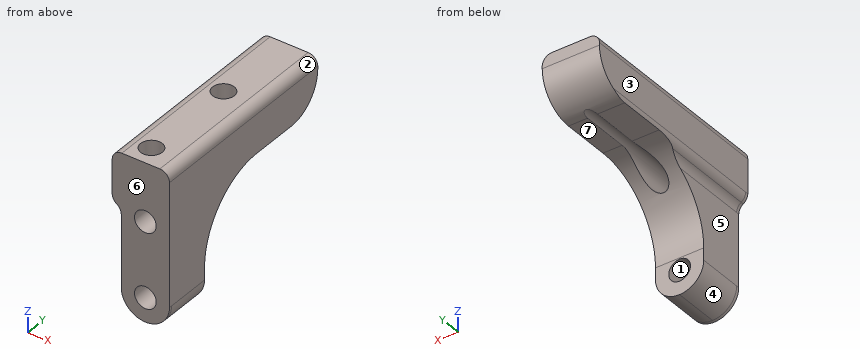
Autodesk Inventor part; units mm, degrees
ref_plane "YZ Plane" through (0, 0, 0) normal (1, 0, 0) x (0, 1, 0)
ref_plane "XZ Plane" through (0, 0, 0) normal (0, 1, 0) x (-1, 0, 0)
ref_plane "XY Plane" through (0, 0, 0) normal (0, 0, 1) x (1, 0, 0)
sketch "スケッチ1" plane through (0, 0, 0) normal (0, 0, 1) x (1, 0, 0)
  line L0 (0, 0) -> (25.5, 0)
  line L1 (25.5, 0) -> (25.5, 41.76)
  line L2 (25.5, 41.76) -> (0, 41.76)
  line L3 (0, 41.76) -> (0, 0)
  line L4 (0, 3) -> (25.5, 3) construction
  line L5 (13.5, 41.76) -> (13.5, 0) construction
  line L6 (12, 41.76) -> (12, 0) construction
  line L7 (12, 7.267) -> (13.5, 7.267)
  line L8 (13.5, 7.267) -> (13.5, 17.554)
  line L9 (13.5, 17.554) -> (12, 17.554)
  line L10 (12, 17.554) -> (12, 7.267)
  line L11 (12, 27.612) -> (13.5, 27.612)
  line L12 (13.5, 27.612) -> (13.5, 37.899)
  line L13 (13.5, 37.899) -> (12, 37.899)
  line L14 (12, 37.899) -> (12, 27.612)
  dimension "d0" = 3
  dimension "d1" = 38.76
  dimension "d2" = 1.5
  dimension "d3" = 12
  dimension "d4" = 25.5
  dimension "d5" = 4.267
  dimension "d6" = 10.287
  dimension "d7" = 10.058
  dimension "d8" = 10.287
  dimension "d11" = 12
extrude "押し出し1" add sketch "スケッチ1" along normal mid plane 7.5
sketch "スケッチ2" plane through (0, 0, -3.75) normal (0, -1, 0) x (1, 0, 0)
  line L0 (25.5, 7.5) -> (0, 7.5)
  line L1 (0, 7.5) -> (25.5, 7.5)
  line L2 (25.5, 7.5) -> (25.5, 2.5)
  line L3 (25.5, -2.5) -> (20.5, -2.5)
  line L4 (0, -2.5) -> (0, 2.5)
  line L5 (25.5, 2.5) -> (0, 2.5) construction
  line L6 (0, 3.75) -> (0, 7.5) construction
  arc A0 (0, 2.5) -> (5, -2.5) centre (5, 2.5) ccw
  line L7 (5, 2.5) -> (5, -2.5) construction
  line L8 (5, 2.5) -> (0, 2.5) construction
  arc A1 (20.5, -2.5) -> (25.5, 2.5) centre (20.5, 2.5) ccw
  line L9 (20.5, 2.5) -> (20.5, -2.5) construction
  line L10 (20.5, 2.5) -> (25.5, 2.5) construction
  line L11 (25.5, 0) -> (25.5, 7.5)
  line L12 (0, 2.5) -> (0, 7.5)
  line L13 (5, -2.5) -> (0, -2.5)
  line L14 (20.5, -2.5) -> (5, -2.5)
  line L15 (25.5, 2.5) -> (25.5, -2.5)
  dimension "d12" = 90
  dimension "d13" = 90
  dimension "d14" = 10
  dimension "d15" = 5
extrude "押し出し2" add sketch "スケッチ2" against normal up to surface (7.267 mm away)
extrude "押し出し3" [suppressed]
ref_plane "作業平面1" through (0, 0, -1.25) normal (0, 0, 1) x (1, 0, 0)
sketch "スケッチ3" plane through (0, 0, 3.75) normal (0, -1, 0) x (1, 0, 0)
  arc A0 (0, -5) -> (5, -10) centre (5, -5) ccw construction
  arc A1 (20.5, -10) -> (25.5, -5) centre (20.5, -5) ccw construction
  circle A2 centre (5, -5) radius 2.25
  circle A3 centre (20.5, -5) radius 2.25
  point P0 (0, -3.75)
  dimension "d20" = 4.5
  dimension "d21" = 4.5
extrude "押し出し4" cut sketch "スケッチ3" against normal up to surface (41.76 mm away)
sketch "スケッチ4" plane through (0.6699, 41.76, -3.75) normal (0, 1, 0) x (1, 0, 0)
  circle A0 centre (19.8301, -2.5) radius 2.25 construction
  circle A1 centre (4.3301, -2.5) radius 2.25 construction
  line L0 (0, 0) -> (24.1603, 0)
  line L1 (19.8301, 0) -> (19.8301, -2.5) construction
  line L2 (17.5801, 0) -> (17.5801, -2.5)
  line L3 (22.0801, -2.5) -> (22.0801, 0)
  arc A2 (22.0801, 0) -> (17.5801, 0) centre (19.8301, 0) ccw
  arc A3 (17.5801, -2.5) -> (22.0801, -2.5) centre (19.8301, -2.5) ccw
  line L4 (4.3301, -0.25) -> (4.3301, -2.5) construction
  line L5 (2.0801, -0.25) -> (2.0801, -2.5)
  line L6 (6.5801, -2.5) -> (6.5801, -0.25)
  arc A4 (6.5801, -0.25) -> (2.0801, -0.25) centre (4.3301, -0.25) ccw
  arc A5 (2.0801, -2.5) -> (6.5801, -2.5) centre (4.3301, -2.5) ccw
  point P0 (-0.6699, -3.75)
  point P1 (19.8301, -1.25)
  point P2 (4.3301, -1.375)
extrude "押し出し5" [suppressed]
sketch "スケッチ5" plane through (12, 7.267, 3.75) normal (1, 0, 0) x (0, 0, -1)
  line L0 (0, 0) -> (7.5, 0) construction
  line L1 (7.5, 10.287) -> (0, 10.287) construction
  line L2 (7.5, 10.287) -> (10, 12.787)
  line L3 (10, 12.787) -> (10, -2.5)
  line L4 (10, -2.5) -> (7.5, 0)
  line L5 (7.5, 0) -> (7.5, 10.287)
  line L6 (10, -7.267) -> (10, 0)
  point P0 (3.75, -7.267)
  dimension "d28" = 135
  dimension "d29" = 135
sketch "スケッチ6" plane through (0, 0, 3.75) normal (0, 0, 1) x (1, 0, 0)
  line L0 (12, 27.612) -> (12, 37.899) construction
  line L1 (12, 37.899) -> (13.5, 37.899) construction
  line L2 (13.5, 37.899) -> (13.5, 27.612) construction
  line L3 (13.5, 27.612) -> (12, 27.612) construction
  line L4 (12, 7.267) -> (12, 17.554) construction
  line L5 (12, 17.554) -> (13.5, 17.554) construction
  line L6 (13.5, 17.554) -> (13.5, 7.267) construction
  line L7 (13.5, 7.267) -> (12, 7.267) construction
  line L8 (0, 0) -> (25.5, 0) construction
  line L9 (25.5, 41.76) -> (0, 41.76) construction
  line L10 (13.625, 27.487) -> (13.625, 38.024)
  line L11 (13.625, 38.024) -> (11.875, 38.024)
  line L12 (11.875, 38.024) -> (11.875, 27.487)
  line L13 (11.875, 27.487) -> (13.625, 27.487)
  line L14 (13.625, 7.142) -> (13.625, 17.679)
  line L15 (13.625, 17.679) -> (11.875, 17.679)
  line L16 (11.875, 17.679) -> (11.875, 7.142)
  line L17 (11.875, 7.142) -> (13.625, 7.142)
  line L18 (0, 41.76) -> (0, 0)
  line L19 (25.5, 0) -> (25.5, 41.76)
  dimension "d32" = 0.125
  dimension "d33" = 0.125
extrude "押し出し7" cut sketch "スケッチ6" against normal through all
sketch "スケッチ8" plane through (0, 0, 3.75) normal (0, -1, 0) x (1, 0, 0)
  line L0 (13.625, 0) -> (13.625, -10) construction
  line L1 (0, 0) -> (0, -10)
  line L2 (0, 0) -> (13.625, 0)
  line L3 (13.625, 0) -> (13.625, -10)
  line L4 (13.625, -10) -> (0, -10)
  line L5 (0, -10) -> (0, 0)
  point P0 (0, -3.75)
extrude "押し出し10" cut sketch "スケッチ8" against normal up to surface (41.76 mm away)
sketch "スケッチ9" plane through (25.5, 7.267, -3.75) normal (0, 1, 0) x (1, 0, 0)
  line L0 (-11.875, 2.5) -> (-11.875, 0)
  line L1 (0, 0) -> (-11.875, 0)
  line L2 (0, 0) -> (0, 2.5)
  line L3 (0, 2.5) -> (-11.875, 2.5)
  point P0 (-25.5, -3.75)
extrude "押し出し11" add sketch "スケッチ9" along normal up to surface (34.493 mm away)
sketch "スケッチ10" plane through (25.5, 0, -6.25) normal (0, -1, 0) x (1, 0, 0)
  line L0 (-11.875, 0) -> (0, 0)
  line L1 (-11.875, 0) -> (0, 0)
  line L2 (0, 0) -> (0, -22.5)
  line L3 (0, -22.5) -> (-11.875, -22.5)
  line L4 (-11.875, -22.5) -> (-11.875, 0)
  circle A0 centre (-5, 5) radius 2.25 construction
  line L5 (-5, 5) -> (-5, -17.5) construction
  circle A1 centre (-5, -17.5) radius 2.25
  point P0 (-25.5, 6.25)
  dimension "d46" = 22.5
  dimension "d47" = 5
  dimension "d48" = 5
extrude "押し出し12" add sketch "スケッチ10" against normal up to surface (41.76 mm away)
sketch "スケッチ12" plane through (13.625, 0, 3.75) normal (0, -1, 0) x (1, 0, 0)
  circle A0 centre (6.875, -5) radius 2.25
  point P0 (-13.625, -3.75)
extrude "押し出し14" add sketch "スケッチ12" against normal up to surface (41.76 mm away)
sketch "スケッチ11" plane through (0, 0, 3.75) normal (0, 0, 1) x (1, 0, 0)
  line L0 (22.75, 0) -> (18.25, 0) construction
  line L1 (18.723, 0) -> (18.723, 3.589) construction
  circle A0 centre (18.723, 3.589) radius 2.25
  line L2 (13.625, 41.76) -> (13.625, 0)
  line L3 (18.723, 3.589) -> (18.723, 24.163) construction
  line L4 (18.25, 0) -> (18.25, 41.76) construction
  circle A1 centre (18.723, 24.163) radius 2.25
  point P0 (0, 0)
  dimension "d51" = 4.5
  dimension "d52" = 3.589
  dimension "d53" = 5.098
  dimension "d54" = 20.574
extrude "押し出し13" cut sketch "スケッチ11" against normal blind 7.5
sketch "スケッチ13" plane through (13.625, 0, 3.75) normal (0, -1, 0) x (1, 0, 0)
  circle A0 centre (6.875, -27.5) radius 2.25 construction
  line L0 (6.875, -27.5) -> (6.875, -12) construction
  circle A1 centre (6.875, -12) radius 2.25
  point P0 (-13.625, -3.75)
  dimension "d59" = 15.5
extrude "押し出し15" cut sketch "スケッチ13" against normal up to surface (41.76 mm away)
sketch "スケッチ14" plane through (13.625, 0, 3.75) normal (0, -1, 0) x (1, 0, 0)
  line L0 (2.848, -7.5) -> (7.348, -7.5) construction
  line L1 (2.848, 0) -> (7.348, 0) construction
  line L2 (0, -32.5) -> (0, 0)
  line L3 (0, -32.5) -> (1.875, -32.5)
  line L4 (1.875, -32.5) -> (1.875, -10.5)
  line L5 (1.875, -10.5) -> (0, -10.5)
  line L6 (0, -10.5) -> (0, -32.5)
  circle A0 centre (6.875, -27.5) radius 2.25
  point P0 (-13.625, -3.75)
  dimension "d62" = 3
  dimension "d63" = 5
extrude "押し出し16" cut sketch "スケッチ14" against normal up to surface (41.76 mm away) contours L2 L5 L4 L3
fillet "フィレット4" radius 2 1 edges at (15.5, 20.88, -6.75)
fillet "フィレット5" radius 5 2 edges at (25.5, 20.88, -28.75) (15.5, 20.88, -28.75)
sketch "スケッチ16" plane through (13.625, 41.76, 3.75) normal (0, 1, 0) x (1, 0, 0)
  arc A0 (11.875, 27.5) -> (1.875, 27.5) centre (6.875, 27.5) ccw
  line L0 (1.875, 27.5) -> (1.875, 12.4961)
  arc A1 (0, 10.5) -> (1.875, 12.4961) centre (-0.125, 12.4961) ccw
  line L1 (0, 10.5) -> (0, 0)
  line L2 (11.875, 0) -> (0, 0)
  line L3 (11.875, 27.5) -> (11.875, 0)
  circle A2 centre (6.875, 27.5) radius 2.25
  circle A3 centre (6.875, 12) radius 2.25
  point P0 (-13.625, 3.75)
extrude "押し出し17" add sketch "スケッチ16" along normal blind 7.928
sketch "スケッチ17" plane through (0, 0, 3.75) normal (0, 0, 1) x (1, 0, 0)
  circle A0 centre (18.723, 3.589) radius 2.25 construction
  circle A1 centre (18.723, 24.163) radius 2.25 construction
  line L0 (18.723, 3.589) -> (18.723, 24.163) construction
  line L1 (18.25, 0) -> (18.25, 49.688) construction
  line L2 (18.723, 24.163) -> (18.723, 44.737) construction
  line L3 (18.723, 44.737) -> (18.723, 65.311) construction
  circle A2 centre (18.723, 44.737) radius 2.25
  circle A3 centre (18.723, 65.311) radius 2.25
  point P0 (0, 0)
extrude "押し出し18" cut sketch "スケッチ17" against normal blind 7.5
fillet "フィレット6" radius 2 1 edges at (13.625, 20.88, -6.7539)
fillet "フィレット7" radius 2 2 edges at (13.625, 24.844, 3.75) (25.5, 24.844, 3.75)
sketch "スケッチ18" plane through (25.5, 0, -23.75) normal (1, 0, 0) x (0, 0, -1)
  line L0 (-27.5, 49.688) -> (-27.5, 0)
  line L1 (-27.5, 41.76) -> (-7.75, 41.76)
  line L2 (0, 0) -> (-25.5, 0)
  arc A0 (5, 29.01) -> (-7.75, 41.76) centre (-7.75, 29.01) ccw
  line L3 (-7.75, 29.01) -> (5, 29.01) construction
  line L4 (-7.75, 29.01) -> (-7.75, 41.76) construction
  line L5 (-27.5, 41.76) -> (-27.5, 50.688)
  line L6 (-27.5, 50.688) -> (6, 50.688)
  line L7 (6, 50.688) -> (6, 29.01)
  line L8 (6, 29.01) -> (5, 29.01)
  line L9 (-25.5, 49.688) -> (0, 49.688)
  line L10 (5, 0) -> (5, 49.688) construction
  point P0 (-23.75, 0)
  dimension "d75" = 41.76
  dimension "d76" = 90
  dimension "d77" = 12.75
  dimension "d78" = 1
  dimension "d79" = 6
extrude "押し出し19" cut sketch "スケッチ18" against normal up to surface (11.875 mm away)
sketch "スケッチ19" plane through (20.5, 0, -23.75) normal (0, -1, 0) x (1, 0, 0)
  arc A0 (5, 25.5) -> (3, 27.5) centre (3, 25.5) ccw
  line L0 (-4.875, 27.5) -> (3, 27.5)
  arc A1 (-4.875, 27.5) -> (-6.875, 25.5) centre (-4.875, 25.5) ccw
  line L1 (-6.875, 18.3928) -> (-6.875, 25.5)
  arc A2 (-6.875, 18.3928) -> (-5.9375, 16.6983) centre (-4.875, 18.3928) ccw
  arc A3 (-5, 15.0039) -> (-5.9375, 16.6983) centre (-7, 15.0039) ccw
  line L2 (-5, 15.0039) -> (-5, 0)
  arc A4 (-5, 0) -> (5, 0) centre (0, 0) ccw
  line L3 (5, 0) -> (5, 25.5)
  circle A5 centre (0, 0) radius 2.25
  circle A6 centre (0, 15.5) radius 2.25
  point P0 (-20.5, 23.75)
extrude "押し出し20" add sketch "スケッチ19" along normal blind 0.6
sketch "スケッチ20" plane through (25.5, 41.76, 1.75) normal (1, 0, 0) x (0, 0, -1)
  line L0 (8, 0) -> (30.5, 0)
  line L1 (30.5, 0) -> (30.5, -32.36)
  line L2 (30.5, -32.36) -> (23, -32.36)
  line L3 (8, 0) -> (8, -17.36)
  line L4 (7.1072, 0) -> (7.1072, -42.36)
  arc A0 (8, -17.36) -> (23, -32.36) centre (23, -17.36) ccw
  line L5 (-2, 0) -> (-2, -42.36)
  line L6 (25.5, -42.36) -> (30.5, -42.36)
  line L7 (30.5, -42.36) -> (30.5, -12.75) construction
  line L8 (17.75, 0) -> (0, 0) construction
  point P0 (1.75, -41.76)
  dimension "d84" = 10
  dimension "d85" = 10
  dimension "d86" = 15
extrude "押し出し21" cut sketch "スケッチ20" against normal up to surface (11.875 mm away)
fillet "フィレット8" radius 7.5 1 edges at (16.6513, 41.76, -6.25)
equation "\"d8\" = d6"
equation "\"d11\" = d3"
equation "\"d29\" = d28"
equation "\"d33\" = d32"
equation "\"d48\" = d47"
properties part number "small_gpu_02" material "アルミニウム 6061"
Geometry: final body of the model. Coordinates: model frame, mm. Face numbers are marked on the shaded views. A direction names the side the tool comes from. Give positions to 0.01 mm unless a question says otherwise; leave off trailing zeros. Order: outer loops, then holes, each group sorted by start corner. A loop starts at its lowest first (then second) coordinate and runs counter-clockwise, first axis right, second up. Notation, with made-up numbers: M -37.5,-13 L -21.5,-13 A30 cw -21.5,17 Z; hole C 44.5,-25.75 d5. An arc over 180 degrees is marked long. Answer as CSV lines item,"result". Start each with the question number.
1) Cut plane A-A (y = 8.5). State how many separate pieces and enclosed holes the cut face has, then the cut area to 3 significant figures.
2) Set-up query: the marked faces 5, 6 and 7. Return all of +Z, -Z, +X, -X, +Y, -Y with unobstructed straight access to the full face (end or side cutting, diameter ignored); none if empty.
3) Line query: line 1 (Z direction, x = 20.5, y = 3); line 2 (Z direction, x = 20.5, y = 2); line 3 (Y direction, x = 18, z = -1). Output: solid intervals per line, ascending. Write a range as from..to.
4) First-contact query: P1, Ø4, axis at x = 18.723, y = 24.163, coming from the +Z side; P2, Ø2.5, axis at x = 20.5, z = -23.75, coming from the +Y side; P3, Ø5, axis at x = 18, y = 23.5, coming from the +Z side; P4, Ø1.7, axis at x = 17, y = 30, coming from the -Z side. Flat tips, straight axial feed; report the tip coordinate or a pass-through.
5) Mould query, pull axis Z, two halves, no side actions, for the marked faces 1, 2, 3 and 4. Classes: +Z half, -Z half, draft (parallel to the pull), parting line (faces both ways), or undercut.
6) Cut plane B-B (z = -2.5). Output: boundary loops of the cut face in (x, y) (3 decimals), then the cut area to 3 significant figures.
Findings below:
1,separate pieces,"1"
1,enclosed holes,"2"
1,area,"301 mm²"
2,face 5,"-Z, -X, +Y, -Y"
2,face 6,"+Z, -Z, +X, -X, -Y"
2,face 7,"-Z, +X, -X, +Y"
3,line 1,"z = -28.75..-26, -21.5..-10.5, -6..-3.75"
3,line 2,"z = -28.75..-26, -21.5..-10.5, -6..3.75"
3,line 3,"y = -0.6..1.46, 5.72..22.03, 26.29..41.41"
4,P1,"stops at z = -3.75"
4,P2,"passes through"
4,P3,"stops at z = 3.75"
4,P4,"stops at z = -6.25"
5,face 1,"undercut"
5,face 2,"+Z half"
5,face 3,"draft"
5,face 4,"-Z half"
6,outline,"M 13.625,-0.6 L 25.5,-0.6 L 25.5,40.755 L 13.625,40.755 Z; hole C 18.723,3.589 d4.5; hole C 18.723,24.163 d4.5"
6,area,"459 mm²"
